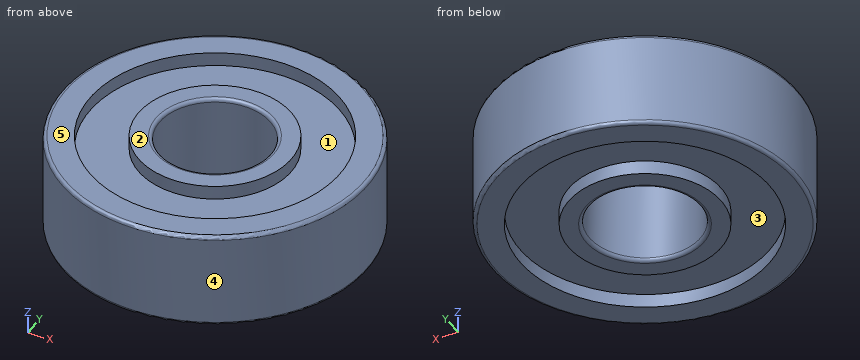
```python
from build123d import *

# Parameters (mm, degrees)
ESQUISSE1_R      = 11
ESQUISSE1_R_2    = 4
EXTRUSION1_DEPTH = 7
CONG_1_R         = 0.25
ESQUISSE2_R      = 9
ESQUISSE2_R_2    = 5.5
EXTRUSION2_DEPTH = 1
EXTRUSION3_START = -1
ESQUISSE3_R      = 9
ESQUISSE3_R_2    = 5.5
EXTRUSION3_DEPTH = 1


with BuildPart() as part:
    # Esquisse1 → Extrusion1 (new body)
    with BuildSketch(Plane.XY):
        Circle(ESQUISSE1_R)
        Circle(ESQUISSE1_R_2, mode=Mode.SUBTRACT)
    extrude(amount=EXTRUSION1_DEPTH)

    # Congé1
    cong_1_edges = [part.edges().sort_by_distance(p)[0] for p in [
        (-11, 0, 0),
        (-11, 0, 7),
        (-4, 0, 0),
        (-4, 0, 7),
    ]]
    fillet(cong_1_edges, radius=CONG_1_R)

    # Esquisse2 → Extrusion2 (cut)
    with BuildSketch(Plane.XY.offset(7)):
        Circle(ESQUISSE2_R)
        Circle(ESQUISSE2_R_2, mode=Mode.SUBTRACT)
    extrude(amount=-EXTRUSION2_DEPTH, mode=Mode.SUBTRACT)

    # Esquisse3 → Extrusion3 (cut)
    with BuildSketch(Plane(origin=(0, 0, 0), x_dir=(-1, 0, 0), z_dir=(0, 0, -1)).offset(EXTRUSION3_START)):
        with Locations(Location((0, 0, 0), (0, 0, 180))):
            Circle(ESQUISSE3_R)
        with Locations(Location((0, 0, 0), (0, 0, 180))):
            Circle(ESQUISSE3_R_2, mode=Mode.SUBTRACT)
    extrude(amount=EXTRUSION3_DEPTH, mode=Mode.SUBTRACT)


solid = part.part
```
Geometry check sheet. Reference: the model listing, model coordinates, mm. Face numbers are marked on the shaded views. A direction names the side the tool comes from. Coordinates: 2 decimals unless noted, no trailing zeros. Write each loop counter-clockwise with the first axis right and the second up, starting at its lowest first coordinate (ties: lowest second). Pieces come first, ordered by that corner, then holes. Notation, with made-up numbers: (-0.75, 73.5) -> (9.25, 73.5) arc R26 ccw to (9.25, 109.5) -> close; hole circle Ø7 at (-20.75, 78.25). An arc over 180 degrees is marked (long way). Use CSV: the item, a comma, the result in double quotes. Start each with the question number.
Item 1: Cross-section at C-C, the plane z = 5.5. Record the cut outline in (x, y), plus the area to 3 significant figures.
Item 2: Thickness scan on line 1 (Y direction, x = 0, z = 6.6); line 2 (X direction, y = 1.25, z = 0.5); line 3 (Y direction, x = 0, z = 2.5). Record the ranges inside material, lowest first.
Item 3: Set-up check for the marked faces 1 and 2: record each of +Z, -Z, +X, -X, +Y, -Y from which the full face is reachable in a straight line by a thin tool's end or side.
Item 4: Mould release check, pull along X, two halves, no side actions. Record for the marked faces 3, 4 and 5: released by +X, released by -X, zero draft, split by the parting line, or undercut.
Item 5: Depth check by flat-ended pin: pin 1 Ø1 at (x, z) = (-2, 1) entering from -Y; pin 2 Ø4 at (x, z) = (-6.5, 2) entering from +Y; pin 3 Ø6.5 at (x, y) = (0, 0) entering from +Z. Enter the tip coordinate at first touch or a pass-through.
Answers:
1,outline,"circle Ø22 at (0, 0); hole circle Ø8 at (0, 0)"
1,area,"330 mm^2"
2,line 1,"-11 to -9, -5.5 to -4, 4 to 5.5, 9 to 11"
2,line 2,"-10.93 to -8.91, -5.36 to -3.8, 3.8 to 5.36, 8.91 to 10.93"
2,line 3,"-11 to -4, 4 to 11"
3,face 1,"+Z"
3,face 2,"+Z, +X, -X, +Y, -Y"
4,face 3,"undercut"
4,face 4,"split by the parting line"
4,face 5,"zero draft"
5,pin 1,"y = -10.9"
5,pin 2,"y = 10.04"
5,pin 3,"through"
